The model under review builds one solid part; all positions refer to its coordinate system, in mm. A direction names the side the tool comes from. Coordinates: 2 decimals unless noted, no trailing zeros. Order: outer loops, then holes, each group sorted by start corner. A loop starts at its lowest first (then second) coordinate and runs counter-clockwise, first axis right, second up. Notation, with made-up numbers: M 31,52.5 L 43,52.5 A17 cw 43,74.5 Z; hole C 79,-13 d8. An arc over 180 degrees is marked long. Write each question's results on one line, items separated by ' | '.
from build123d import *

# Parameters (mm, degrees)
SKETCH1_R           = 7
BOSS_EXTRUDE1_DEPTH = 10


with BuildPart() as part:
    # Sketch1 → Boss-Extrude1 (new body)
    with BuildSketch(Plane(origin=(0, 0, 0), x_dir=(1, 0, 0), z_dir=(0, 1, 0))):
        with BuildLine():
            Line((-42.331013445, 0), (-10.444849334, 26.755668546))
            ThreePointArc((-10.444849334, 26.755668546), (-7.979712665, 54.932309602), (-36.156353721, 57.39744627))
            Line((-36.156353721, 57.39744627), (-61.156353721, 36.419955491))
            Line((-61.156353721, 36.419955491), (-61.156353721, -23.580044509))
            Line((-61.156353721, -23.580044509), (9.843646279, -94.580044509))
            ThreePointArc((9.843646279, -94.580044509), (31.279693612, -95.296110549), (31.518421727, -73.849435172))
            Line((31.518421727, -73.849435172), (-42.331013445, 0))
        make_face()
        with Locations(Location((20.911820009, -84.456036889, 0), (0, 0, 270))):
            Circle(SKETCH1_R, mode=Mode.SUBTRACT)
        with Locations(Location((-9.088179991, -54.456036889, 0), (0, 0, 270))):
            Circle(SKETCH1_R, mode=Mode.SUBTRACT)
        with Locations(Location((-39.088179991, -24.456036889, 0), (0, 0, 270))):
            Circle(SKETCH1_R, mode=Mode.SUBTRACT)
    extrude(amount=BOSS_EXTRUDE1_DEPTH)


solid = part.part
1) For faces 1 (the flat face through (-4.89, 4.93, 37.44)), 2 (the flat face through (-61.156, 5, -7)), list the 3-axis set-ups (+Z, -Z, +X, -X, +Y, -Y) from which the entire face can be reached by the end or side of a thin tool; tool diameter is ignored.
Solutions:
face 1: +X, +Y, -Y | face 2: +Z, -Z, -X, +Y, -Y
2) For pin 1 (2 mm diameter, centred on x = 4.5, y = 4, fed in from +Z); pin 2 (3 mm diameter, centred on x = -47, y = 7.5, fed in from -Z), all flat-tipped, find the tip position at first contact; note any pin that passes through.
Solutions:
pin 1: z = 90.24 | pin 2: z = -49.56
3) Take a section at B-B on z = 53.5. State the section outline as (x, y) points, plus the area to 3 significant figures.
Solutions:
outline: M -31.24,0 L -16.02,0 L -16.02,10 L -31.24,10 Z; M -2.15,0 L 11.17,0 L 11.17,10 L -2.15,10 Z | area: 285 mm2
4) Take a section at A-A on x = -26. State the section outline as (y, z) points.
Solutions:
outline: M 0,-61.89 L 10,-61.89 L 10,-13.7 L 0,-13.7 Z; M 0,16.33 L 10,16.33 L 10,58.74 L 0,58.74 Z
5) To check wall thickness, follow line 1 along Z through (x, y) = (-42, 9.5); line 2 along Z through (x, y) = (-37.5, 8.5); line 3 along X through (y, z) = (9.5, 56). State the ranges of each line that lie inside material, in increasing order.
Solutions:
line 1: -52.49 to -0.28, 0.33 to 18.09, 30.82 to 42.74 | line 2: -56.27 to -4.05, 4.83 to 17.64, 31.27 to 47.24 | line 3: -28.74 to -15.92, -2.26 to 13.67
6) Take a section at C-C on x = -5. State the section outline as (y, z) points.
Solutions:
outline: M 0,-50.14 L 10,-50.14 L 10,-34.01 L 0,-34.01 Z; M 0,37.33 L 10,37.33 L 10,48.77 L 0,48.77 Z; M 0,60.14 L 10,60.14 L 10,79.74 L 0,79.74 Z
7) Take a section at D-D on y = 7.5. State the section outline as (x, z) points, plus the area to 3 significant figures.
Solutions:
outline: M -61.16,-36.42 L -36.16,-57.4 A20 ccw -10.44,-26.76 L -42.33,0 L 31.52,73.85 A15 ccw long 9.84,94.58 L -61.16,23.58 Z; hole C -39.09,24.46 d14; hole C -9.09,54.46 d14; hole C 20.91,84.46 d14 | area: 5,650 mm2
